The figure shows three views and two pictorial views of one solid part (mm, origin at its lowest corner). Answer the questions. A direction names the side the tool comes from. Coordinates: 2 decimals unless noted, no trailing zeros. Order: outer loops, then holes, each group sorted by start corner. A loop starts at its lowest first (then second) coordinate and runs counter-clockwise, first axis right, second up. Notation, with made-up numbers: (9, -5.75) -> (55, -5.75) arc R11 cw to (55, 8.25) -> close; hole circle Ø7 at (77.5, 60.25). An arc over 180 degrees is marked (long way). Return JSON: item names as keys, results as strings.
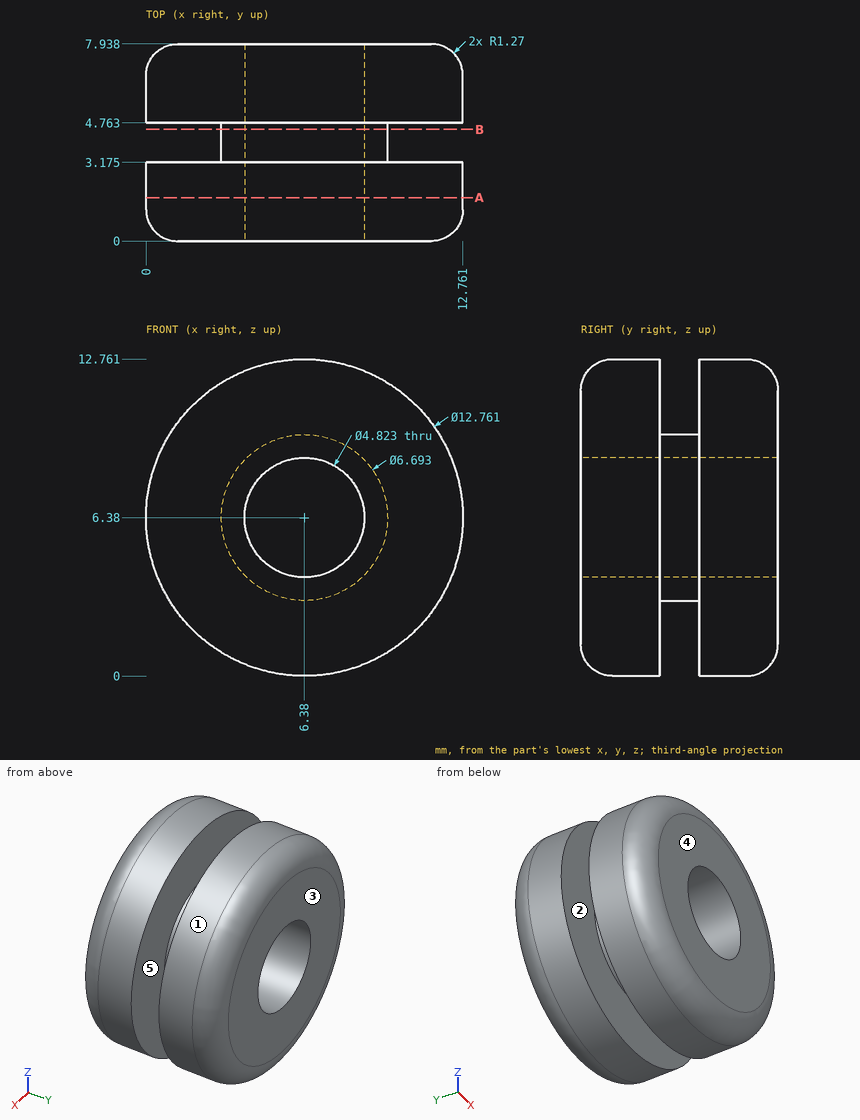
Item 1: Find the intervals of material crossed by probe 1 along Y at (x, z) = (9.75, 6.75) (1 decimal); probe 2 along X at (y, z) = (2.5, 6.5); probe 3 along X at (y, z) = (1.25, 6), in increasing order.
Answer list:
{"probe 1": "0 to 3.2, 4.8 to 7.9", "probe 2": "0 to 3.97, 8.79 to 12.76", "probe 3": "0.01 to 4, 8.76 to 12.75"}
Item 2: Flat-ended cylindrical pins translate along their axes: pin 1 (4 mm diameter, centred on x = 4.5, z = 5.5, fed in from +Y); pin 2 (1.5 mm diameter, centred on x = 2.5, y = 5.5, fed in from +Z); pin 3 (1 mm diameter, centred on x = 7, y = 4, fed in from +Z) (1 decimal). Find the tip coordinate at first contact, or state that the pin passes through.
Answer list:
{"pin 1": "y = 7.94", "pin 2": "z = 11.94", "pin 3": "z = 9.7"}
Item 3: Determine the mould class of the marked faces 1, 2 and 3 for opening direction Y: pulls with the +Y half, pulls with the -Y half, needs draft (parallel to the pull), parting line crosses it, or undercut.
Answer list:
{"face 1": "needs draft", "face 2": "undercut", "face 3": "pulls with the +Y half"}
Item 4: The part is cut by section B-B on y = 4.5. Determine the outline of the cut face in (x, z).
Answer list:
{"outline": "circle Ø6.69 at (6.38, 6.38); hole circle Ø4.82 at (6.38, 6.38)"}
Item 5: Which of the six approach directions +Z, -Z, +X, -X, +Y, -Y give full straight-line access (tool end or side, diameter ignored) to the marked faces 4 and 5?
Answer list:
{"face 4": "+Z, -Z, +X, -X, -Y", "face 5": "none"}
Item 6: The part is cut by section A-A on y = 1.75. Determine the outline of the cut face in (x, z).
Answer list:
{"outline": "circle Ø12.76 at (6.38, 6.38); hole circle Ø4.82 at (6.38, 6.38)"}
